Geometry check sheet. Reference: the model listing, model coordinates, mm. A direction names the side the tool comes from. Coordinates: 2 decimals unless noted, no trailing zeros. Loops run counter-clockwise (first coordinate to the right, second up) from the corner with the lowest first, then second, coordinate; pieces in that order, holes last.
from build123d import *

# Parameters (mm, degrees)
SKETCH1_R                         = 21.59
SKETCH1_R_2                       = 6.35
BOSS_EXTRUDE1_DEPTH               = 0.7874
SKETCH2_W                         = 5.6
SKETCH2_H                         = 13
SKETCH2_W_2                       = 13
SKETCH2_H_2                       = 5.6
FACE_BOARD_CONNECTORS_DEPTH       = 3
SKETCH3_W                         = 13
SKETCH3_H                         = 5.6
BOTTOM_FACE_BOARD_CONNECTOR_DEPTH = 3
PROGRAMMING_CONNECTOR_DEPTH       = 3
SKETCH5_W                         = 2.8
SKETCH5_H                         = 2.95
I2C_TRANSLATOR_DEPTH              = 1.3
SKETCH6_W                         = 5
SKETCH6_H                         = 3
ACCELEROMETER_DEPTH               = 1
SKETCH7_W                         = 2
SKETCH7_H                         = 1
BOSS_EXTRUDE7_DEPTH               = 0.45
BOSS_EXTRUDE8_DEPTH               = 1.2
SKETCH9_W                         = 2.69
SKETCH9_H                         = 6.5
BOSS_EXTRUDE9_DEPTH               = 2.69


with BuildPart() as part:
    # Sketch1 → Boss-Extrude1 (new body)
    with BuildSketch(Plane(origin=(0, 0, 0), x_dir=(1, 0, 0), z_dir=(0, 1, 0))):
        Circle(SKETCH1_R)
        Circle(SKETCH1_R_2, mode=Mode.SUBTRACT)
    extrude(amount=BOSS_EXTRUDE1_DEPTH)

    # Sketch2 → Face Board Connectors (add)
    with BuildSketch(Plane(origin=(0, 0.7874, 0), x_dir=(1, 0, 0), z_dir=(0, 1, 0))):
        with Locations((-16.25, 0)):
            Rectangle(SKETCH2_W, SKETCH2_H)
        with Locations((0, 16.25)):
            Rectangle(SKETCH2_W_2, SKETCH2_H_2)
        with Locations((0, -16.25)):
            Rectangle(SKETCH2_W_2, SKETCH2_H_2)
        with Locations((16.25, 0)):
            Rectangle(SKETCH2_W, SKETCH2_H)
    extrude(amount=FACE_BOARD_CONNECTORS_DEPTH)

    # Sketch3 → Bottom Face Board Connector (add)
    with BuildSketch(Plane.XZ):
        with Locations((0, 16.25)):
            Rectangle(SKETCH3_W, SKETCH3_H)
    extrude(amount=BOTTOM_FACE_BOARD_CONNECTOR_DEPTH)

    # Sketch4 → Programming Connector (add)
    with BuildSketch(Plane(origin=(0, 0.7874, 0), x_dir=(1, 0, 0), z_dir=(0, 1, 0))):
        Polygon((-18.00114237, 11.920024051), (-14.112055073, 8.030936755), (-8.030936755, 14.112055073), (-11.920024051, 18.00114237), align=None)
    extrude(amount=PROGRAMMING_CONNECTOR_DEPTH)

    # Sketch5 → I2C Translator (add)
    with BuildSketch(Plane(origin=(0, 0.7874, 0), x_dir=(1, 0, 0), z_dir=(0, 1, 0))):
        with Locations((-11.276551559, -11.592117418)):
            Rectangle(SKETCH5_W, SKETCH5_H)
    extrude(amount=I2C_TRANSLATOR_DEPTH)

    # Sketch6 → Accelerometer (add)
    with BuildSketch(Plane(origin=(0, 0.7874, 0), x_dir=(1, 0, 0), z_dir=(0, 1, 0))):
        with Locations((12.21999094, -10.814372721)):
            Rectangle(SKETCH6_W, SKETCH6_H)
    extrude(amount=ACCELEROMETER_DEPTH)

    # Sketch7 → Boss-Extrude7 (add)
    with BuildSketch(Plane(origin=(0, 0.7874, 0), x_dir=(1, 0, 0), z_dir=(0, 1, 0))):
        with Locations((10.71999094, -14.443290742)):
            Rectangle(SKETCH7_W, SKETCH7_H)
    extrude(amount=BOSS_EXTRUDE7_DEPTH)

    # Sketch8 → Boss-Extrude8 (add)
    with BuildSketch(Plane.XZ):
        Polygon((-9.844993145, -16.845350279), (-2.844636011, -9.844993145), (-9.844993145, -2.844636011), (-16.845350279, -9.844993145), align=None)
    extrude(amount=BOSS_EXTRUDE8_DEPTH)

    # Sketch9 → Boss-Extrude9 (add)
    with BuildSketch(Plane.XZ):
        with Locations((-10.391917908, 8.664203432)):
            Rectangle(SKETCH9_W, SKETCH9_H)
    extrude(amount=BOSS_EXTRUDE9_DEPTH)


solid = part.part
(1) Sectioned sample at A-A on z = 0. Record the cut outline in (x, y), and give its area (3 significant figures).
Findings:
outline: (-21.59, 0) - (-6.35, 0) - (-6.35, 0.79) - (-13.45, 0.79) - (-13.45, 3.79) - (-19.05, 3.79) - (-19.05, 0.79) - (-21.59, 0.79) - close; (6.35, 0) - (21.59, 0) - (21.59, 0.79) - (19.05, 0.79) - (19.05, 3.79) - (13.45, 3.79) - (13.45, 0.79) - (6.35, 0.79) - close
area: 57.6 mm2
(2) Sectioned sample at C-C on x = 5. Record the cut outline in (y, z).
Findings:
outline: (-3, 13.45) - (0, 13.45) - (0, 3.91) - (0.79, 3.91) - (0.79, 13.45) - (3.79, 13.45) - (3.79, 19.05) - (0.79, 19.05) - (0.79, 21) - (0, 21) - (0, 19.05) - (-3, 19.05) - close; (0, -21) - (0.79, -21) - (0.79, -19.05) - (3.79, -19.05) - (3.79, -13.45) - (0.79, -13.45) - (0.79, -3.91) - (0, -3.91) - close
(3) Sectioned sample at D-D on x = -7.5. Record the cut outline in (y, z), and give its area (3 significant figures).
Findings:
outline: (-1.2, -14.5) - (0, -14.5) - (0, -20.25) - (0.79, -20.25) - (0.79, 20.25) - (0, 20.25) - (0, -5.19) - (-1.2, -5.19) - close
area: 43.1 mm2
(4) Scan lines: L1, parallel to Z at x = 0, y = 0.65; L2, parallel to Z at x = -3, y = 1.5. Record each from-to range of solid material in increasing order.
Findings:
L1: z = -21.59 to -6.35, 6.35 to 21.59
L2: z = -19.05 to -13.45, 13.45 to 19.05
(5) Draft check along Z on faces 4 (the flat face through (0, 2, 13.45)), 5 (the flat face through (-13, -1, -6)), 6 (the cylindrical face through (-15.913, 0.388, -14.592)), 7 (the flat face through (9.72, 1, 11)). Enter one of: +Z half, -Z half, draft (parallel to the pull), parting line (faces both ways), or undercut.
Findings:
face 4: undercut
face 5: undercut
face 6: parting line
face 7: draft
(6) Sectioned sample at B-B on x = 0. Record the cut outline in (y, z), and give its area (3 significant figures).
Findings:
outline: (-3, 13.45) - (0, 13.45) - (0, 6.35) - (0.79, 6.35) - (0.79, 13.45) - (3.79, 13.45) - (3.79, 19.05) - (0.79, 19.05) - (0.79, 21.59) - (0, 21.59) - (0, 19.05) - (-3, 19.05) - close; (0, -21.59) - (0.79, -21.59) - (0.79, -19.05) - (3.79, -19.05) - (3.79, -13.45) - (0.79, -13.45) - (0.79, -6.35) - (0, -6.35) - close
area: 74.4 mm2
(7) Access from +Z, -Z, +X, -X, +Y, -Y to the whole of each face (thin tool, end or side, straight path). Record for faces 1 (the flat face through (-11, 1, 10.117)), 2 (the flat face through (6.5, -1, 16)), 3 (the flat face through (-9.047, -1, 9)).
Findings:
face 1: -X, +Y
face 2: +Z, -Z, +X, -Y
face 3: +Z, +X, -Y
(8) Gauge pin test, flat ends, axial feed: pin 1 Ø0.9 at (y, z) = (3, -0.5) entering from -X; pin 2 Ø3 at (x, z) = (3, -6.5) entering from -Y; pin 3 Ø15.5 at (x, z) = (-11.5, -7.5) entering from -Y. Record the tip position at first contact, or that the pin passes through.
Findings:
pin 1: stops at x = -19.05
pin 2: stops at y = 0
pin 3: stops at y = -1.2
